```python
from build123d import *

# Parameters (mm, degrees)
F0_W      = 51.8160052598
F0_H      = 89.0015969053
F0_R      = 9.7547897259
F1_DEPTH  = 27.432
F2_W      = 25.1459991559
F2_H      = 15.1513946929
F2_W_2    = 24.2315987125
F3_DEPTH  = 18.288
F4_W      = 25.7555991411
F4_H      = 13.7160010636
F4_W_2    = 23.3171992004
F5_DEPTH  = 16.256
F6_W      = 89.0015969053
F6_H      = 17.8308002651
F7_DEPTH  = 4.064
F8_W      = 24.9466653913
F8_H      = 17.8308002651
F8_W_2    = 24.7357338667
F9_DEPTH  = 25.4
F10_W     = 28.8035981357
F10_H     = 16.9163998216
F10_W_2   = 29.4131976552
F10_H_2   = 17.8308002651
F11_DEPTH = 25.4


with BuildPart() as f1:
    # F0 (on Top) → F1 (new body)
    with BuildSketch(Plane.XY):
        with Locations((1.5240013599, 7.7724005096)):
            Rectangle(F0_W, F0_H)
        with Locations((1.5240013599, 7.7724005096)):
            Circle(F0_R, mode=Mode.SUBTRACT)
    extrude(amount=F1_DEPTH)

    # F2 (on face) → F3 (join)
    with BuildSketch(Plane.YZ.offset(27.4320039898)):
        with Locations((-24.1553983651, 45.0302423907)):
            Rectangle(F2_W, F2_H)
        Polygon((-11.5823987871, 37.4545450442), (-36.7283979431, 37.4545450442), (-36.7283979431, 0), (52.2731989622, 0), (52.2731989622, 37.4545450442), (28.0416002497, 37.4545450442), align=None)
        with Locations((40.157399606, 45.0302423907)):
            Rectangle(F2_W_2, F2_H)
    extrude(amount=F3_DEPTH)

    # F4 (on face) → F5 (join)
    with BuildSketch(Plane(origin=(-24.3840012699, 0, 0), x_dir=(0, -1, 0), z_dir=(-1, 0, 0))):
        with Locations((-39.3953993917, 39.0144009143)):
            Rectangle(F4_W, F4_H)
        Polygon((-26.5175998211, 32.1564003825), (-52.2731989622, 32.1564003825), (-52.2731989622, 0), (36.7283979431, 0), (36.7283979431, 32.1564003825), (13.4111987427, 32.1564003825), align=None)
        with Locations((25.0697983429, 39.0144009143)):
            Rectangle(F4_W_2, F4_H)
    extrude(amount=F5_DEPTH)

    # F6 (on face) → F7 (join)
    with BuildSketch(Plane.YZ.offset(45.7200039898)):
        with Locations((7.7724005096, 8.9154001325)):
            Rectangle(F6_W, F6_H)
    extrude(amount=F7_DEPTH)

    # F8 (on face) → F9 (join)
    with BuildSketch(Plane.YZ.offset(49.7840039898)):
        with Locations((-24.2550652474, 8.9154001325)):
            Rectangle(F8_W, F8_H)
        with Locations((39.9053320289, 8.9154001325)):
            Rectangle(F8_W_2, F8_H)
    extrude(amount=F9_DEPTH)

    # F10 (on face) → F11 (join)
    with BuildSketch(Plane(origin=(-40.6400012699, 0, 0), x_dir=(0, -1, 0), z_dir=(-1, 0, 0))):
        with Locations((-37.8713998944, 8.4581999108)):
            Rectangle(F10_W, F10_H)
        with Locations((22.0217991155, 8.9154001325)):
            Rectangle(F10_W_2, F10_H_2)
    extrude(amount=F11_DEPTH)


solid = f1.part
```
Geometry: final body of the model. Coordinates: model frame, mm. A direction names the side the tool comes from. Give positions to 0.01 mm unless a question says otherwise; leave off trailing zeros. Order: outer loops, then holes, each group sorted by start corner. A loop starts at its lowest first (then second) coordinate and runs counter-clockwise, first axis right, second up. Notation, with made-up numbers: (24, 74) -> (78, 74) arc R14 ccw to (78, 90) -> close; hole circle Ø5 at (65.25, 60.25). An arc over 180 degrees is marked (long way). Write each question's results on one line, items separated by ' | '. Start each with the question number.
1) Section A-A (x = -47.5). Return loops of the section in (y, z).
2) Line query: line 1 (X direction, y = -28.5, z = 31); line 2 (Y direction, x = -51.5, z = 13.5); line 3 (Y direction, x = 53, z = 17). Output: solid intervals per line, ascending. Write a range as from..to.
3) First-contact query: pin 1 (18 mm diameter, centred on x = -31.5, y = -22, fed in from +Z); pin 2 (7.5 mm diameter, centred on x = -48, y = 34, fed in from +Z); pin 3 (10 mm diameter, centred on y = 20, z = 45.5, fed in from -X); pin 4 (13 mm diameter, centred on x = -36, y = 1.5, fed in from +Z). Flat tips, straight axial feed; report the tip coordinate or a pass-through.
4) Section C-C (y = 45). Return loops of the section in (x, z).
5) Section B-B (x = 38). Return loops of the section in (y, z), then the cut area to 3 significant figures.
6) Section D-D (z = 7). Return loops of the section in (x, y), then the cut area to 3 significant figures.
7) Set-up query: faces 1 (the flat face through (1, 18, 27.432)), 2 (the flat face through (45.72, 7, 32)), 3 (the flat face through (-32, -13.411, 39)). Return all of +Z, -Z, +X, -X, +Y, -Y with unobstructed straight access to the full face (end or side cutting, diameter ignored); none if empty.
Calculated:
1) outline: (-36.73, 0) -> (-7.32, 0) -> (-7.32, 17.83) -> (-36.73, 17.83) -> close; (23.47, 0) -> (52.27, 0) -> (52.27, 16.92) -> (23.47, 16.92) -> close
2) line 1: -40.64..-24.38, 27.43..45.72 | line 2: -36.73..-7.32, 23.47..52.27 | line 3: -36.73..-11.78, 27.54..52.27
3) pin 1: z = 45.87 | pin 2: z = 16.92 | pin 3: through | pin 4: z = 32.16
4) outline: (-66.04, 0) -> (75.18, 0) -> (75.18, 17.83) -> (45.72, 17.83) -> (45.72, 52.61) -> (27.43, 52.61) -> (27.43, 27.43) -> (-24.38, 27.43) -> (-24.38, 45.87) -> (-40.64, 45.87) -> (-40.64, 16.92) -> (-66.04, 16.92) -> close
5) outline: (-36.73, 0) -> (52.27, 0) -> (52.27, 52.61) -> (28.04, 52.61) -> (28.04, 37.45) -> (-11.58, 37.45) -> (-11.58, 52.61) -> (-36.73, 52.61) -> close | area: 4,080 mm2
6) outline: (-66.04, -36.73) -> (75.18, -36.73) -> (75.18, -11.78) -> (49.78, -11.78) -> (49.78, 27.54) -> (75.18, 27.54) -> (75.18, 52.27) -> (-66.04, 52.27) -> (-66.04, 23.47) -> (-40.64, 23.47) -> (-40.64, -7.32) -> (-66.04, -7.32) -> close; hole circle Ø19.51 at (1.52, 7.77) | area: 10,500 mm2
7) face 1: +Z, +Y, -Y | face 2: +Z, +X, +Y, -Y | face 3: +Z, -X
